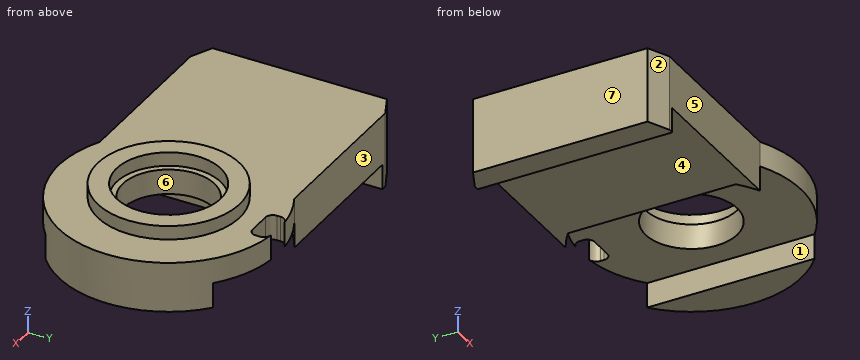
```python
from build123d import *

# Parameters (mm, degrees)
SKETCH_310_R           = 3.65
EXTRUDE_1379_DEPTH     = 4
CUT_EXTRUDE_1435_DEPTH = 2
CUT_EXTRUDE_2054_DEPTH = 2
EXTRUDE_2114_DEPTH     = 2
SKETCH_4_R             = 5.65
SKETCH_4_R_2           = 4.15
EXTRUDE_4_DEPTH        = 1.1


with BuildPart() as part:
    # Sketch 310 → Extrude 1379 (new body)
    with BuildSketch(Plane.XY):
        with BuildLine():
            ThreePointArc((-4.062019202, -7.75), (8.75, 0), (-4.062019202, 7.75))
            Line((-4.062019202, 7.75), (-17.062019202, 7.75))
            Line((-17.062019202, 7.75), (-18.75, 6.953209217))
            Line((-18.75, 6.953209217), (-18.75, -6.953209217))
            Line((-18.75, -6.953209217), (-17.062019202, -7.75))
            Line((-17.062019202, -7.75), (-4.062019202, -7.75))
        make_face()
        Circle(SKETCH_310_R, mode=Mode.SUBTRACT)
    extrude(amount=EXTRUDE_1379_DEPTH)

    # Sketch 1_3 → Cut-Extrude 1435 (cut)
    with BuildSketch(Plane.XY):
        with BuildLine():
            Line((5.65, 6.681317235), (5.65, -6.681317235))
            ThreePointArc((5.65, -6.681317235), (0, -8.75), (-5.65, -6.681317235))
            Line((-5.65, -6.681317235), (-5.65, 6.681317235))
            ThreePointArc((-5.65, 6.681317235), (0, 8.75), (5.65, 6.681317235))
        make_face()
    extrude(amount=CUT_EXTRUDE_1435_DEPTH, mode=Mode.SUBTRACT)

    # Sketch 1681 → Cut-Extrude 2054 (cut)
    with BuildSketch(Plane(origin=(0, 0, 2), x_dir=(-1, 0, 0), z_dir=(0, 0, -1))):
        with BuildLine():
            Line((-1.5, 7.78), (-1.5, 8.082233602))
            ThreePointArc((-1.5, 8.082233602), (-1.341523495, 8.496233679), (-0.947109471, 8.6985909))
            ThreePointArc((-0.947109471, 8.6985909), (0, 8.75), (0.947109471, 8.6985909))
            ThreePointArc((0.947109471, 8.6985909), (1.341523495, 8.496233679), (1.5, 8.082233602))
            Line((1.5, 8.082233602), (1.5, 7.78))
            ThreePointArc((1.5, 7.78), (1.330121933, 7.369878067), (0.92, 7.2))
            Line((0.92, 7.2), (-0.92, 7.2))
            ThreePointArc((-0.92, 7.2), (-1.330121933, 7.369878067), (-1.5, 7.78))
        make_face()
    extrude(amount=-CUT_EXTRUDE_2054_DEPTH, mode=Mode.SUBTRACT)

    # Sketch 1_5 → Extrude 2114 (add)
    with BuildSketch(Plane.XY):
        Polygon((-16.65, -7.75), (-16.65, 7.75), (-17.062019202, 7.75), (-18.75, 6.953209217), (-18.75, -6.953209217), (-17.062019202, -7.75), align=None)
    extrude(amount=-EXTRUDE_2114_DEPTH)

    # Sketch 4 → Extrude 4 (add)
    with BuildSketch(Plane.XY.offset(4)):
        Circle(SKETCH_4_R)
        Circle(SKETCH_4_R_2, mode=Mode.SUBTRACT)
    extrude(amount=EXTRUDE_4_DEPTH)


solid = part.part
```
Geometry check sheet. Reference: the model listing, model coordinates, mm. Face numbers are marked on the shaded views. A direction names the side the tool comes from. Coordinates: 2 decimals unless noted, no trailing zeros. Loops run counter-clockwise (first coordinate to the right, second up) from the corner with the lowest first, then second, coordinate; pieces in that order, holes last.
Item 1: Release check for a two-part mould opening along X. For the marked faces 5, 6 and 7 record: released by +X, released by -X, zero draft, split by the parting line, or undercut.
Item 2: Sectioned sample at C-C, the plane z = 3.25. Record the boundary of the cut face in (x, y).
Item 3: Sectioned sample at D-D, the plane z = -0.5. Record the boundary of the cut face in (x, y).
Item 4: Sectioned sample at A-A, the plane x = 0. Record the boundary of the cut face in (y, z), then the cut area to 3 significant figures.
Item 5: Sectioned sample at B-B, the plane y = 0. Record the boundary of the cut face in (x, z).
Item 6: Access from +Z, -Z, +X, -X, +Y, -Y to the whole of each face (thin tool, end or side, straight path). Record for the marked faces 1, 2, 3 and 4.
Item 7: Go/stop test with flat-tipped pins: pin 1 Ø2 at (x, z) = (-6, 1) entering from -Y; pin 2 Ø3.5 at (x, y) = (-2.5, -4) entering from -Z; pin 3 Ø3.5 at (x, y) = (6.5, -0.5) entering from -Z; pin 4 Ø5 at (x, y) = (-1.5, -2) entering from +Z. Record where each tip stops, or that it passes through.
Item 8: Thickness scan on line 1 (X direction, y = 0, z = 3); line 2 (Y direction, x = 0, z = 4.6); line 3 (X direction, y = -1.25, z = -0.75). Record the ranges inside material, lowest first.
Check result:
1. face 5: zero draft
1. face 6: undercut
1. face 7: released by -X
2. outline: (-18.75, -6.95) - (-17.06, -7.75) - (-4.06, -7.75) arc R8.75 ccw (long way) to (0.95, 8.7) arc R0.62 cw to (1.5, 8.08) - (1.5, 7.78) arc R0.58 cw to (0.92, 7.2) - (-0.92, 7.2) arc R0.58 cw to (-1.5, 7.78) - (-1.5, 8.08) arc R0.62 cw to (-0.95, 8.7) arc R8.75 ccw to (-4.06, 7.75) - (-17.06, 7.75) - (-18.75, 6.95) - close; hole circle Ø7.3 at (0, 0)
3. outline: (-18.75, -6.95) - (-17.06, -7.75) - (-16.65, -7.75) - (-16.65, 7.75) - (-17.06, 7.75) - (-18.75, 6.95) - close
4. outline: (-8.75, 2) - (-3.65, 2) - (-3.65, 4) - (-4.15, 4) - (-4.15, 5.1) - (-5.65, 5.1) - (-5.65, 4) - (-8.75, 4) - close; (3.65, 2) - (7.2, 2) - (7.2, 4) - (5.65, 4) - (5.65, 5.1) - (4.15, 5.1) - (4.15, 4) - (3.65, 4) - close
4. area: 20.6 mm2
5. outline: (-18.75, -2) - (-16.65, -2) - (-16.65, 0) - (-5.65, 0) - (-5.65, 2) - (-3.65, 2) - (-3.65, 4) - (-4.15, 4) - (-4.15, 5.1) - (-5.65, 5.1) - (-5.65, 4) - (-18.75, 4) - close; (3.65, 2) - (5.65, 2) - (5.65, 0) - (8.75, 0) - (8.75, 4) - (5.65, 4) - (5.65, 5.1) - (4.15, 5.1) - (4.15, 4) - (3.65, 4) - close
6. face 1: -Z, +Y, -Y
6. face 2: +Z, -Z, -X, -Y
6. face 3: +Z, -Z, -X, +Y
6. face 4: -Z, +X, +Y, -Y
7. pin 1: stops at y = -7.75
7. pin 2: stops at z = 2
7. pin 3: stops at z = 0
7. pin 4: stops at z = 5.1
8. line 1: x = -18.75 to -3.65, 3.65 to 8.75
8. line 2: y = -5.65 to -4.15, 4.15 to 5.65
8. line 3: x = -18.75 to -16.65
